CAD build for the part. Positions are in the model's coordinates, mm. Coordinates: 2 decimals unless noted, no trailing zeros. Order: outer loops, then holes, each group sorted by start corner. A loop starts at its lowest first (then second) coordinate and runs counter-clockwise, first axis right, second up. Notation, with made-up numbers: (74.5, 89.5) -> (83.5, 89.5) arc R17 ccw to (83.5, 121.5) -> close; hole circle Ø4 at (36.5, 71). An arc over 180 degrees is marked (long way). Use one line per item in the form item = value. Start each with the question number.
from build123d import *

# Parameters (mm, degrees)
SKETCH_1_W                     = 40
SKETCH_1_H                     = 24
SKETCH_1_R                     = 5.8
SKETCH_1_R_2                   = 1.7
BEARING_RETAINER_40X24X2_DEPTH = 2


with BuildPart() as part:
    # 草图1 → Bearing_retainer_40x24x2 (new body)
    with BuildSketch(Plane.XY):
        Rectangle(SKETCH_1_W, SKETCH_1_H)
        Circle(SKETCH_1_R, mode=Mode.SUBTRACT)
        with Locations((-14, 0)):
            Circle(SKETCH_1_R_2, mode=Mode.SUBTRACT)
        with Locations((14, 0)):
            Circle(SKETCH_1_R_2, mode=Mode.SUBTRACT)
    extrude(amount=BEARING_RETAINER_40X24X2_DEPTH)


solid = part.part
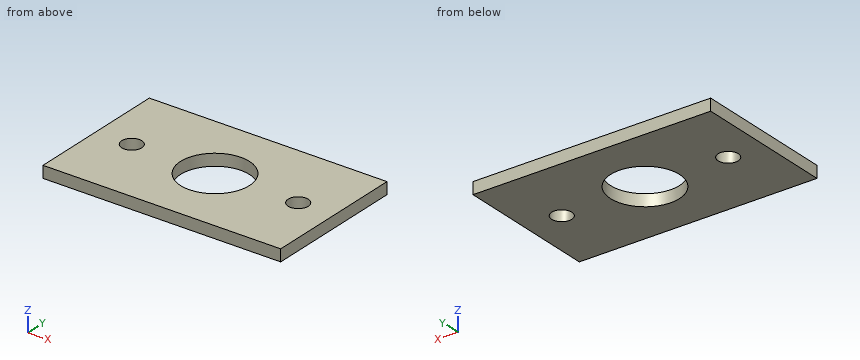
1) Cut at A-A on x = -14. Give the cut face in (y, z), then the cut area to 3 significant figures.
2) Cut at D-D on z = 1.25. Give the cut face in (x, y).
3) Cut at C-C on y = 0. Give the cut face in (x, z), then the cut area to 3 significant figures.
4) Drop a flat-ended pin along its axis: P1, Ø5.5, axis at x = 14, y = 0, coming from the -Z side. Give the stop position or say it passes through.
5) Probe L1, parallel to Y at x = -14, z = 0.4; L2, parallel to X at y = 0.5, z = 0.35; L3, parallel to X at y = -0.25, z = 0.2. List the from-to ranges inside material, lowest first.
6) Cut at B-B on y = -4. Give the cut face in (x, z).
Values follow:
q1.outline = (-12, 0) -> (-1.7, 0) -> (-1.7, 2) -> (-12, 2) -> close; (1.7, 0) -> (12, 0) -> (12, 2) -> (1.7, 2) -> close
q1.area = 41.2 mm^2
q2.outline = (-20, -12) -> (20, -12) -> (20, 12) -> (-20, 12) -> close; hole circle Ø3.4 at (-14, 0); hole circle Ø11.6 at (0, 0); hole circle Ø3.4 at (14, 0)
q3.outline = (-20, 0) -> (-15.7, 0) -> (-15.7, 2) -> (-20, 2) -> close; (-12.3, 0) -> (-5.8, 0) -> (-5.8, 2) -> (-12.3, 2) -> close; (5.8, 0) -> (12.3, 0) -> (12.3, 2) -> (5.8, 2) -> close; (15.7, 0) -> (20, 0) -> (20, 2) -> (15.7, 2) -> close
q3.area = 43.2 mm^2
q4.P1 = 0
q5.L1 = -12 to -1.7, 1.7 to 12
q5.L2 = -20 to -15.62, -12.38 to -5.78, 5.78 to 12.38, 15.62 to 20
q5.L3 = -20 to -15.68, -12.32 to -5.79, 5.79 to 12.32, 15.68 to 20
q6.outline = (-20, 0) -> (-4.2, 0) -> (-4.2, 2) -> (-20, 2) -> close; (4.2, 0) -> (20, 0) -> (20, 2) -> (4.2, 2) -> close
